The listing builds one solid part. Answer for the finished solid, in the listing's coordinates (mm). A direction names the side the tool comes from. Round coordinates to 2 decimals unless told otherwise and drop trailing zeros. Order: outer loops, then holes, each group sorted by start corner. A loop starts at its lowest first (then second) coordinate and runs counter-clockwise, first axis right, second up. Notation, with made-up numbers: (30, 21.25) -> (89, 21.25) arc R27 cw to (89, 41.25) -> close; hole circle Ø3 at (7.5, 68.5). An arc over 180 degrees is marked (long way). Return JSON: item names as keys, results as strings. Group by question number.
(1) The part is cut by section C-C (y = -63.5). Determine the outline of the cut face in (x, z), plus the area to 3 significant figures.
(2) Which of the six approach directions +Z, -Z, +X, -X, +Y, -Y give full straight-line access (tool end or side, diameter ignored) to faces 1 (the face through (-14, -60, 3)), 2 (the face through (-13.703, -50.462, 1.479))?
(3) Consider line 1 (X direction, y = -60.5, z = 1.1); line 2 (Y direction, x = -41, z = 1.65); line 3 (X direction, y = -48, z = 2.55). Determine where each line is inside the solid, lowest interval first. Write a range as [from, to].
(4) The part is cut by section D-D (x = -22). Determine the outline of the cut face in (y, z).
(5) The part is cut by section A-A (x = -11). Determine the outline of the cut face in (y, z), plus the area to 3 significant figures.
(6) This flat-tipped pin is pushed along its axis until it touches: pin 1 (1 mm diameter, centred on y = -69, z = 1, fed in from -X). Where does it stop, or does it pass through?
(7) The part is cut by section B-B (z = 1.15). Determine the outline of the cut face in (x, y).
from build123d import *

# Parameters (mm, degrees)
SKETCH_1_R          = 18
LASHENA_DEPTH       = 3
CUT_EXTRUDEA_DEPTH  = 3
WWW_KYTOOL_CN_COUNT = 16
SKETCH_3_R          = 1.5
CUT_EXTRUDE_2_DEPTH = 10
SKETCH_4_R          = 1.5
CUT_EXTRUDE_3_DEPTH = 10
EXTRUDE_START       = -3
EXTRUDE_1_DEPTH     = 3
SKETCH_6_R          = 1.5
CUT_EXTRUDE_4_DEPTH = 3
SKETCH_7_R          = 35
CUT_EXTRUDE_5_DEPTH = 3


with BuildPart() as part:
    # Sketch 1 → LaShenA (new body)
    with BuildSketch(Plane.XY):
        Circle(SKETCH_1_R)
    extrude(amount=LASHENA_DEPTH)

    # SketchA → Cut-ExtrudeA (cut)
    with BuildSketch(Plane.XY.offset(3)):
        with BuildLine():
            ThreePointArc((0.423212707, 13.493364703), (0, 13.5), (-0.423212707, 13.493364703))
            ThreePointArc((-0.423212707, 13.493364703), (-0.952770902, 13.685686791), (-1.20440395, 14.18977059))
            add(Edge.make_bspline(
                [(-1.20440395, 14.18977059), (-1.226562505, 14.455224305), (-1.213843633, 14.773889884), (-1.273675597, 15.110607864), (-1.299119688, 15.21139578), (-1.321432077, 15.29109757), (-1.349914152, 15.382250837), (-1.385146673, 15.484587535), (-1.427834192, 15.597770763), (-1.478623281, 15.721446817), (-1.538159915, 15.855229004), (-1.607069773, 15.998703507), (-1.685962928, 16.151428337), (-1.775430978, 16.312934487), (-1.876046532, 16.482726463), (-1.98836201, 16.660283053), (-2.112908684, 16.845058076), (-2.250195688, 17.036481179), (-2.400709063, 17.233958676), (-2.56491084, 17.43687441), (-2.743238138, 17.644590662), (-2.936102365, 17.856449073), (-3.14388814, 18.07177164), (-3.447378451, 18.368492697), (-3.689495989, 18.585006365), (-3.858042439, 18.727457792)],
                knots=[0.122308221, 0.122308221, 0.122308221, 0.122308221, 0.250610689, 0.276296194, 0.287604067, 0.300967916, 0.316387742, 0.333863545, 0.353395324, 0.37498308, 0.398626813, 0.424326522, 0.452082207, 0.48189387, 0.513761509, 0.547685125, 0.583664717, 0.621700286, 0.661791832, 0.703939355, 0.748142854, 0.79440233, 0.842717782, 0.893089212, 1, 1, 1, 1], degree=3))
            ThreePointArc((-3.858042439, 18.727457792), (0, 19.120726106), (3.858042439, 18.727457792))
            add(Edge.make_bspline(
                [(1.20440395, 14.18977059), (1.226562505, 14.455224305), (1.213843633, 14.773889884), (1.273675597, 15.110607864), (1.299119688, 15.21139578), (1.321432077, 15.29109757), (1.349914152, 15.382250837), (1.385146673, 15.484587535), (1.427834192, 15.597770763), (1.478623281, 15.721446817), (1.538159915, 15.855229004), (1.607069773, 15.998703507), (1.685962928, 16.151428337), (1.775430978, 16.312934487), (1.876046532, 16.482726463), (1.98836201, 16.660283053), (2.112908684, 16.845058076), (2.250195688, 17.036481179), (2.400709063, 17.233958676), (2.56491084, 17.43687441), (2.743238138, 17.644590662), (2.936102365, 17.856449073), (3.14388814, 18.07177164), (3.447378451, 18.368492697), (3.689495989, 18.585006365), (3.858042439, 18.727457792)],
                knots=[0.122308221, 0.122308221, 0.122308221, 0.122308221, 0.250610689, 0.276296194, 0.287604067, 0.300967916, 0.316387742, 0.333863545, 0.353395324, 0.37498308, 0.398626813, 0.424326522, 0.452082207, 0.48189387, 0.513761509, 0.547685125, 0.583664717, 0.621700286, 0.661791832, 0.703939355, 0.748142854, 0.79440233, 0.842717782, 0.893089212, 1, 1, 1, 1], degree=3))
            ThreePointArc((1.20440395, 14.18977059), (0.952770902, 13.685686791), (0.423212707, 13.493364703))
        make_face()
    cut_extrudea = extrude(amount=-CUT_EXTRUDEA_DEPTH, mode=Mode.SUBTRACT)

    # www.KYTool.cn: Cut-ExtrudeA ×16 about axis
    www_kytool_cn_axis = Axis((0, 0, -80.9), (0, 0, 1))
    for i in range(1, WWW_KYTOOL_CN_COUNT):
        add(cut_extrudea.rotate(www_kytool_cn_axis, i * 360 / WWW_KYTOOL_CN_COUNT), mode=Mode.SUBTRACT)

    # Sketch 3 → Cut-Extrude 2 (cut)
    with BuildSketch(Plane(origin=(0, 0, 0), x_dir=(-1, 0, 0), z_dir=(0, 0, -1))):
        Circle(SKETCH_3_R)
    extrude(amount=-CUT_EXTRUDE_2_DEPTH, mode=Mode.SUBTRACT)

    # Sketch 4 → Cut-Extrude 3 (cut)
    with BuildSketch(Plane(origin=(0, 0, 0), x_dir=(-1, 0, 0), z_dir=(0, 0, -1))):
        with Locations((5, 0)):
            Circle(SKETCH_4_R)
        with Locations((0, -5)):
            Circle(SKETCH_4_R)
        with Locations((-5, 0)):
            Circle(SKETCH_4_R)
        with Locations((0, 5)):
            Circle(SKETCH_4_R)
    extrude(amount=-CUT_EXTRUDE_3_DEPTH, mode=Mode.SUBTRACT)

    # Sketch 5 → Extrude 1 (add)
    with BuildSketch(Plane.XY.offset(3).offset(EXTRUDE_START)):
        with BuildLine():
            ThreePointArc((-4.772689561, -12.628199965), (-4.970068688, -12.551829239), (-5.166226337, -12.472373689))
            Line((-5.166226337, -12.472373689), (-6.888301783, -16.629831585))
            Line((-6.888301783, -16.629831585), (-4.283870626, -17.147885152))
            add(Edge.make_bspline(
                [(-4.317465956, -13.570544057), (-4.398578859, -13.824271023), (-4.532277602, -14.113812327), (-4.605856468, -14.447795879), (-4.620919058, -14.550648803), (-4.630805653, -14.632822238), (-4.639374492, -14.727936493), (-4.645986446, -14.835966176), (-4.649861667, -14.95686965), (-4.650267444, -15.090567568), (-4.646458993, -15.236949875), (-4.637699901, -15.395873694), (-4.623257392, -15.567164141), (-4.602405419, -15.750614308), (-4.574425345, -15.945985545), (-4.538607339, -16.153007717), (-4.494251555, -16.371379528), (-4.440669352, -16.600768877), (-4.377184493, -16.840813269), (-4.322953121, -17.024128059), (-4.290370833, -17.127506691), (-4.283870626, -17.147885152)],
                knots=[0.122308221, 0.122308221, 0.122308221, 0.122308221, 0.250610689, 0.276296194, 0.287604067, 0.300967916, 0.316387742, 0.333863545, 0.353395324, 0.37498308, 0.398626813, 0.424326522, 0.452082207, 0.48189387, 0.513761509, 0.547685125, 0.583664717, 0.621700286, 0.661791832, 0.703939355, 0.714301745, 0.714301745, 0.714301745, 0.714301745], degree=3))
            ThreePointArc((-4.317465956, -13.570544057), (-4.35704006, -13.008535554), (-4.772689561, -12.628199965))
        make_face()
        with BuildLine():
            ThreePointArc((-4.159224889, -17.512876643), (-5.541381013, -17.125802068), (-6.888301783, -16.629831585))
            Line((-6.888301783, -16.629831585), (-17.226084522, -67.950540756))
            ThreePointArc((-17.226084522, -67.950540756), (-13.675837107, -68.753075978), (-10.088719252, -69.370250979))
            Line((-10.088719252, -69.370250979), (0, -18))
            Line((0, -18), (-5.56603723, -45.982358781))
            Line((-5.56603723, -45.982358781), (-9.010188121, -45.297274573))
            Line((-9.010188121, -45.297274573), (-3.511625796, -17.654135047))
            ThreePointArc((-3.511625796, -17.654135047), (-3.836075605, -17.58648697), (-4.159224889, -17.512876643))
        make_face()
        with BuildLine():
            Line((-4.283870626, -17.147885152), (-6.888301783, -16.629831585))
            ThreePointArc((-6.888301783, -16.629831585), (-5.541381013, -17.125802068), (-4.159224889, -17.512876643))
            add(Edge.make_bspline(
                [(-4.283870626, -17.147885152), (-4.26264249, -17.214436374), (-4.222189787, -17.336486596), (-4.179302136, -17.457699367), (-4.159224889, -17.512876643)],
                knots=[0.714301745, 0.714301745, 0.714301745, 0.714301745, 0.748142854, 0.776587965, 0.776587965, 0.776587965, 0.776587965], degree=3))
        make_face()
        with BuildLine():
            ThreePointArc((-10.088719252, -69.370250979), (-13.675837107, -68.753075978), (-17.226084522, -67.950540756))
            Line((-17.226084522, -67.950540756), (-18.736412238, -75.448385449))
            ThreePointArc((-18.736412238, -75.448385449), (-15.166327168, -76.24627552), (-11.562659331, -76.875333623))
            Line((-11.562659331, -76.875333623), (-10.088719252, -69.370250979))
        make_face()
        with BuildLine():
            Line((-18.736412238, -75.448385449), (-17.226084522, -67.950540756))
            ThreePointArc((-17.226084522, -67.950540756), (-28.498456938, -64.045701878), (-38.945489094, -58.286043408))
            Line((-38.945489094, -58.286043408), (-43.190045675, -64.638471246))
            ThreePointArc((-43.190045675, -64.638471246), (-31.43143504, -71.102580134), (-18.736412238, -75.448385449))
        make_face()
        with BuildLine():
            add(Edge.make_bspline(
                [(-1.20440395, -14.18977059), (-1.226562505, -14.455224305), (-1.213843633, -14.773889884), (-1.273675597, -15.110607864), (-1.299119688, -15.21139578), (-1.321432077, -15.29109757), (-1.349914152, -15.382250837), (-1.385146673, -15.484587535), (-1.427834192, -15.597770763), (-1.478623281, -15.721446817), (-1.538159915, -15.855229004), (-1.607069773, -15.998703507), (-1.685962928, -16.151428337), (-1.775430978, -16.312934487), (-1.876046532, -16.482726463), (-1.98836201, -16.660283053), (-2.112908684, -16.845058076), (-2.250195688, -17.036481179), (-2.400709063, -17.233958676), (-2.52096385, -17.38256601), (-2.590627249, -17.465606711), (-2.604431157, -17.481946433)],
                knots=[0.122308221, 0.122308221, 0.122308221, 0.122308221, 0.250610689, 0.276296194, 0.287604067, 0.300967916, 0.316387742, 0.333863545, 0.353395324, 0.37498308, 0.398626813, 0.424326522, 0.452082207, 0.48189387, 0.513761509, 0.547685125, 0.583664717, 0.621700286, 0.661791832, 0.703939355, 0.714301745, 0.714301745, 0.714301745, 0.714301745], degree=3))
            Line((-2.604431157, -17.481946433), (0, -18))
            Line((0, -18), (0, -13.5))
            ThreePointArc((0, -13.5), (-0.211632359, -13.498341074), (-0.423212707, -13.493364703))
            ThreePointArc((-0.423212707, -13.493364703), (-0.952770902, -13.685686791), (-1.20440395, -14.18977059))
        make_face()
        with BuildLine():
            Line((0, -18), (-2.604431157, -17.481946433))
            add(Edge.make_bspline(
                [(-2.604431157, -17.481946433), (-2.649511447, -17.535308089), (-2.733591469, -17.632587212), (-2.819600611, -17.728160816), (-2.859264998, -17.771454743)],
                knots=[0.714301745, 0.714301745, 0.714301745, 0.714301745, 0.748142854, 0.776587965, 0.776587965, 0.776587965, 0.776587965], degree=3))
            ThreePointArc((-2.859264998, -17.771454743), (-1.434192217, -17.942772715), (0, -18))
        make_face()
        with BuildLine():
            ThreePointArc((-2.859264998, -17.771454743), (-3.185985461, -17.71579794), (-3.511625796, -17.654135047))
            Line((-3.511625796, -17.654135047), (-9.010188121, -45.297274573))
            Line((-9.010188121, -45.297274573), (-5.56603723, -45.982358781))
            Line((-5.56603723, -45.982358781), (0, -18))
            ThreePointArc((0, -18), (-1.434192217, -17.942772715), (-2.859264998, -17.771454743))
        make_face()
    extrude(amount=EXTRUDE_1_DEPTH)

    # Sketch 6 → Cut-Extrude 4 (cut)
    with BuildSketch(Plane(origin=(0, 0, 0), x_dir=(-1, 0, 0), z_dir=(0, 0, -1))):
        with Locations((14.241593507, -71.597325469)):
            Circle(SKETCH_6_R)
        with Locations((11.705419321, -58.847116824)):
            Circle(SKETCH_6_R)
    extrude(amount=-CUT_EXTRUDE_4_DEPTH, mode=Mode.SUBTRACT)

    # Sketch 7 → Cut-Extrude 5 (cut)
    with BuildSketch(Plane(origin=(0, 0, 0), x_dir=(-1, 0, 0), z_dir=(0, 0, -1))):
        Circle(SKETCH_7_R)
    extrude(amount=-CUT_EXTRUDE_5_DEPTH, mode=Mode.SUBTRACT)


solid = part.part
Answer below:
{
 "1": {"outline": "(-42.43, 0) -> (-29.69, 0) -> (-29.69, 3) -> (-42.43, 3) -> close; (-16.33, 0) -> (-8.94, 0) -> (-8.94, 3) -> (-16.33, 3) -> close", "area": "60.4 mm²"},
 "2": {"face 1": "+Z, +X, -X, +Y, -Y", "face 2": "+Z, -Z, +Y"},
 "3": {"line 1": "x = [-40.42, -35.41], [-15.73, -8.35]", "line 2": "y = [-66.05, -61.36]", "line 3": "x = [-13.21, -5.89]"},
 "4": {"outline": "(-74.56, 0) -> (-66.56, 0) -> (-66.56, 3) -> (-74.56, 3) -> close"},
 "5": {"outline": "(-74.01, 0) -> (-60.17, 0) -> (-60.17, 3) -> (-74.01, 3) -> close; (-57.52, 0) -> (-37.04, 0) -> (-37.04, 3) -> (-57.52, 3) -> close", "area": "103 mm²"},
 "6": {"pin 1": "stops at x = -36.76"},
 "7": {"outline": "(-43.19, -64.64) arc R77.74 ccw to (-11.56, -76.88) -> (-3.31, -34.84) arc R35 cw to (-10.28, -33.46) -> (-17.23, -67.95) arc R70.1 cw to (-38.95, -58.29) -> close; hole circle Ø3 at (-14.24, -71.6); hole circle Ø3 at (-11.71, -58.85)"}
}
